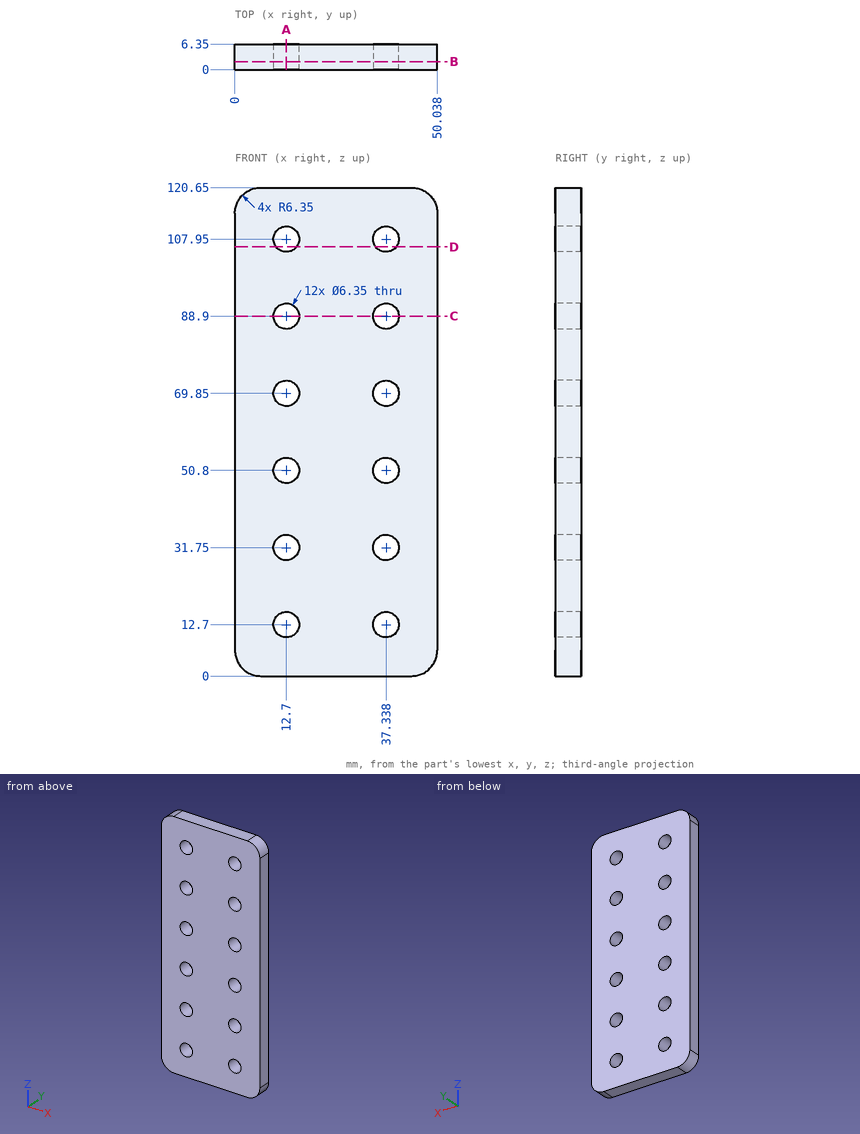
Source: three-view drawing plus pictorial views. Frame: mm from the lowest corner of the part. Coordinates: 2 decimals unless noted, no trailing zeros. Write each loop counter-clockwise with the first axis right and the second up, starting at its lowest first coordinate (ties: lowest second). Pieces come first, ordered by that corner, then holes. Notation, with made-up numbers: (-14.75, -16.5) - (-3.75, -16.5) arc R11 cw to (-3.75, -6.5) - close; hole circle Ø2 at (66, 47.25). An arc over 180 degrees is marked (long way). Answer as a JSON object with one key per item and string values.
Q1. Section query D-D, the plane z = 106. Output: boundary loops of the cut face in (x, y).
Ans:
{"outline": "(0, 0) - (10.19, 0) - (10.19, 6.35) - (0, 6.35) - close; (15.21, 0) - (34.83, 0) - (34.83, 6.35) - (15.21, 6.35) - close; (39.84, 0) - (50.04, 0) - (50.04, 6.35) - (39.84, 6.35) - close"}
Q2. Section query A-A, the plane x = 12.7. Output: boundary loops of the cut face in (y, z) (3 decimals).
Ans:
{"outline": "(0, 0) - (6.35, 0) - (6.35, 9.525) - (0, 9.525) - close; (0, 15.875) - (6.35, 15.875) - (6.35, 28.575) - (0, 28.575) - close; (0, 34.925) - (6.35, 34.925) - (6.35, 47.625) - (0, 47.625) - close; (0, 53.975) - (6.35, 53.975) - (6.35, 66.675) - (0, 66.675) - close; (0, 73.025) - (6.35, 73.025) - (6.35, 85.725) - (0, 85.725) - close; (0, 92.075) - (6.35, 92.075) - (6.35, 104.775) - (0, 104.775) - close; (0, 111.125) - (6.35, 111.125) - (6.35, 120.65) - (0, 120.65) - close"}
Q3. Section query B-B, the plane y = 2. State how many separate pieces and enclosed holes the cut face has, plus the area to 3 significant figures.
Ans:
{"separate pieces": "1", "enclosed holes": "12", "area": "5,620 mm2"}
Q4. First-contact query: pin 1 Ø4 at (x, z) = (12.7, 31.75) entering from +Y. Flat tip, straight axial feed; report the tip coordinate or a pass-through.
Ans:
{"pin 1": "passes through"}
Q5. Section query C-C, the plane z = 88.9. Output: boundary loops of the cut face in (x, y) (3 decimals), plus the area to 3 significant figures.
Ans:
{"outline": "(0, 0) - (9.525, 0) - (9.525, 6.35) - (0, 6.35) - close; (15.875, 0) - (34.163, 0) - (34.163, 6.35) - (15.875, 6.35) - close; (40.513, 0) - (50.038, 0) - (50.038, 6.35) - (40.513, 6.35) - close", "area": "237 mm2"}
Q6. Material intervals for line 1 (X direction, y = 1.5, z = 88.9) (3 decimals); line 2 (X direction, y = 3.5, z = 86.5); line 3 (X direction, y = 5.25, z = 115.5), sorted ascending. Write a range as [from, to].
Ans:
{"line 1": "x = [0, 9.525], [15.875, 34.163], [40.513, 50.038]", "line 2": "x = [0, 10.62], [14.78, 35.26], [39.42, 50.04]", "line 3": "x = [0.11, 49.92]"}
